```python
from build123d import *

# Parameters (mm, degrees)
SKETCH1_W                      = 98
SKETCH1_H                      = 99
MAIN_BODY_DEPTH                = 1
SKETCH2_R                      = 1.75
FRONTBACKBOLTHOLES_DEPTH       = 2
SKETCH3_R                      = 1.75
SIDEBOLTHOLES_DEPTH            = 2
SKETCH7_W                      = 9
SKETCH7_H                      = 13.5
CUT_EXTRUDE3_DEPTH             = 2
FILLET1_R                      = 4
BOSS_EXTRUDE4_DEPTH            = 2
CAMERAVIEWHOLE_DEPTH           = 4
M3X0_5_TAPPED_HOLE1_D          = 2.5
M3X0_5_TAPPED_HOLE1_DEPTH      = 7.5
M3X0_5_TAPPED_HOLE1_TIP        = 0.751075774
SKETCH16_R                     = 1
WIREPASSTHROUGHS_DEPTH         = 4
SKETCH17_R                     = 2.05
NOTSUREIFNEEDPASSTHROUGH_DEPTH = 4


with BuildPart() as part:
    # Sketch1 → Main Body (new body)
    with BuildSketch(Plane.XY):
        with Locations((49, 49.5)):
            Rectangle(SKETCH1_W, SKETCH1_H)
    extrude(amount=MAIN_BODY_DEPTH)

    # Sketch2 → FrontBackBoltHoles (cut, through all)
    with BuildSketch(Plane.XY.offset(1)):
        with Locations((4, 82)):
            Circle(SKETCH2_R)
        with Locations((94, 82)):
            Circle(SKETCH2_R)
        with Locations((94, 17)):
            Circle(SKETCH2_R)
        with Locations((4, 17)):
            Circle(SKETCH2_R)
    extrude(amount=-FRONTBACKBOLTHOLES_DEPTH, mode=Mode.SUBTRACT)

    # Sketch3 → SideBoltHoles (cut, through all)
    with BuildSketch(Plane.XY.offset(1)):
        with Locations((21, 96)):
            Circle(SKETCH3_R)
        with Locations((77, 96)):
            Circle(SKETCH3_R)
        with Locations((77, 3)):
            Circle(SKETCH3_R)
        with Locations((21, 3)):
            Circle(SKETCH3_R)
    extrude(amount=-SIDEBOLTHOLES_DEPTH, mode=Mode.SUBTRACT)

    # Sketch7 → Cut-Extrude3 (cut, through all)
    with BuildSketch(Plane.XY.offset(1)):
        with Locations((4.5, 92.25)):
            Rectangle(SKETCH7_W, SKETCH7_H)
        with Locations((93.5, 92.25)):
            Rectangle(SKETCH7_W, SKETCH7_H)
        with Locations((93.5, 6.75)):
            Rectangle(SKETCH7_W, SKETCH7_H)
        with Locations((4.5, 6.75)):
            Rectangle(SKETCH7_W, SKETCH7_H)
    extrude(amount=-CUT_EXTRUDE3_DEPTH, mode=Mode.SUBTRACT)

    # Fillet1
    fillet1_edges = [part.edges().sort_by_distance(p)[0] for p in [
        (89, 85.5, 0.5),
        (9, 13.5, 0.5),
        (89, 13.5, 0.5),
        (9, 85.5, 0.5),
    ]]
    fillet(fillet1_edges, radius=FILLET1_R)

    # Sketch15 → Boss-Extrude4 (add)
    with BuildSketch(Plane(origin=(0, 0, 0), x_dir=(-1, 0, 0), z_dir=(0, 0, -1))):
        with BuildLine():
            Line((-22.5, 93.5), (-75.5, 93.5))
            ThreePointArc((-75.5, 93.5), (-86.106601718, 89.106601718), (-90.5, 78.5))
            Line((-90.5, 78.5), (-90.5, 20.5))
            ThreePointArc((-90.5, 20.5), (-86.106601718, 9.893398282), (-75.5, 5.5))
            Line((-75.5, 5.5), (-22.5, 5.5))
            ThreePointArc((-22.5, 5.5), (-11.893398282, 9.893398282), (-7.5, 20.5))
            Line((-7.5, 20.5), (-7.5, 78.5))
            ThreePointArc((-7.5, 78.5), (-11.893398282, 89.106601718), (-22.5, 93.5))
        make_face()
        with BuildLine():
            Line((-35.5, 90.5), (-62.5, 90.5))
            ThreePointArc((-62.5, 90.5), (-80.17766953, 83.17766953), (-87.5, 65.5))
            Line((-87.5, 65.5), (-87.5, 33.5))
            ThreePointArc((-87.5, 33.5), (-80.17766953, 15.82233047), (-62.5, 8.5))
            Line((-62.5, 8.5), (-35.5, 8.5))
            ThreePointArc((-35.5, 8.5), (-17.82233047, 15.82233047), (-10.5, 33.5))
            Line((-10.5, 33.5), (-10.5, 65.5))
            ThreePointArc((-10.5, 65.5), (-17.82233047, 83.17766953), (-35.5, 90.5))
        make_face(mode=Mode.SUBTRACT)
    extrude(amount=BOSS_EXTRUDE4_DEPTH)

    # Sketch10 → CameraViewHole (cut, through all)
    with BuildSketch(Plane.XY.offset(1)):
        with BuildLine():
            Line((40, 35.5), (40, 63.5))
            ThreePointArc((40, 63.5), (49, 72.5), (58, 63.5))
            Line((58, 63.5), (58, 35.5))
            ThreePointArc((58, 35.5), (49, 26.5), (40, 35.5))
        make_face()
    extrude(amount=-CAMERAVIEWHOLE_DEPTH, mode=Mode.SUBTRACT)

    # M3x0.5 Tapped Hole1
    with Locations(Plane.XY.offset(1)):
        with Locations((84, 14.5), (14, 14.5), (14, 84.5), (84, 84.5)):
            Hole(M3X0_5_TAPPED_HOLE1_D / 2, depth=M3X0_5_TAPPED_HOLE1_DEPTH)
            with Locations((0, 0, -(M3X0_5_TAPPED_HOLE1_DEPTH + M3X0_5_TAPPED_HOLE1_TIP / 2))):  # 118° drill point
                Cone(0, M3X0_5_TAPPED_HOLE1_D / 2, M3X0_5_TAPPED_HOLE1_TIP, mode=Mode.SUBTRACT)

    # Sketch16 → WirePassthroughs (cut, through all)
    with BuildSketch(Plane.XY.offset(1)):
        with Locations((27.787, 28.287)):
            Circle(SKETCH16_R)
        with Locations((38.393, 38.893)):
            Circle(SKETCH16_R)
        with Locations((59.607, 60.107)):
            Circle(SKETCH16_R)
        with Locations((70.213, 70.713)):
            Circle(SKETCH16_R)
    extrude(amount=-WIREPASSTHROUGHS_DEPTH, mode=Mode.SUBTRACT)

    # Sketch17 → NotSureIfNeedPassthrough (cut, through all)
    with BuildSketch(Plane.XY.offset(1)):
        with Locations((49, 23.5)):
            Circle(SKETCH17_R)
        with Locations((23, 49.5)):
            Circle(SKETCH17_R)
        with Locations((49, 75.5)):
            Circle(SKETCH17_R)
        with Locations((75, 49.5)):
            Circle(SKETCH17_R)
    extrude(amount=-NOTSUREIFNEEDPASSTHROUGH_DEPTH, mode=Mode.SUBTRACT)


solid = part.part
```
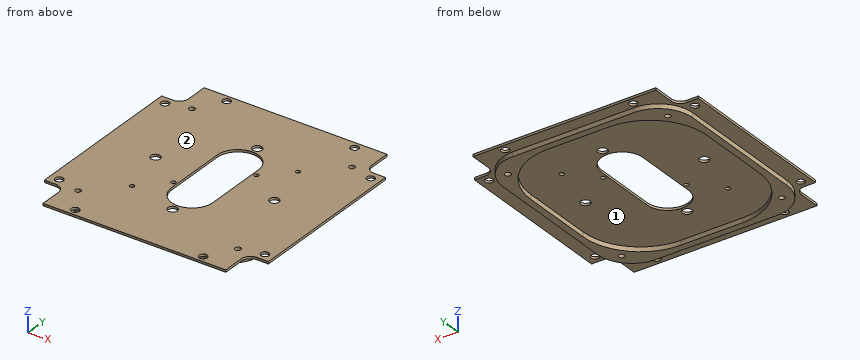
Geometry check sheet. Reference: the model listing, model coordinates, mm. Face numbers are marked on the shaded views. Round coordinates to 2 decimals unless told otherwise and drop trailing zeros. Order: outer loops, then holes, each group sorted by start corner. A loop starts at its lowest first (then second) coordinate and runs counter-clockwise, first axis right, second up. Notation, with made-up numbers: (44, 46.5) -> (57, 46.5) arc R28 cw to (57, 83.5) -> close; hole circle Ø11 at (35.5, -31.75). An arc over 180 degrees is marked (long way). Return JSON: item names as keys, results as strings. Group by question number.
Q1. Section check B-B, the plane x = 49. Record the boundary of the cut face in (y, z).
Q2. Section check A-A, the plane y = 96. Record the boundary of the cut face in (x, z), plus the area to 3 significant figures.
Q3. Material ranges on probe 1 along X at (y, z) = (82, 0.7); probe 2 along Y at (x, z) = (49, 0.2); probe 3 along Y at (x, z) = (4, 0.4), recorded low to high. Write a range as from..to.
Q4. Gauge pin test, flat ends, axial feed: pin 1 (2.5 mm diameter, centred on x = 23, y = 49.5, fed in from -Z); pin 2 (1.6 mm diameter, centred on x = 45.5, z = -1, fed in from -Y); pin 3 (2 mm diameter, centred on x = 63, y = 30.5, fed in from -Z); pin 4 (0.8 mm diameter, centred on x = 2.5, z = 0.5, fed in from +Y). Record the tip position at first contact, or that the pin passes through.
Q5. Section check C-C, the plane y = 49.5. Record the boundary of the cut face in (x, z), plus the area to 3 significant figures.
Q6. Section check D-D, the plane x = 84. Record the boundary of the cut face in (y, z), plus the area to 3 significant figures.
Q7. Release check for a two-part mould opening along X. For the marked faces 1 and 2 record: released by +X, released by -X, zero draft, split by the parting line, or undercut.
Numbers:
{
 "1": {"outline": "(0, 0) -> (5.5, 0) -> (5.5, -2) -> (8.5, -2) -> (8.5, 0) -> (21.45, 0) -> (21.45, 1) -> (0, 1) -> close; (25.55, 0) -> (26.5, 0) -> (26.5, 1) -> (25.55, 1) -> close; (72.5, 0) -> (73.45, 0) -> (73.45, 1) -> (72.5, 1) -> close; (77.55, 0) -> (90.5, 0) -> (90.5, -2) -> (93.5, -2) -> (93.5, 0) -> (99, 0) -> (99, 1) -> (77.55, 1) -> close"},
 "2": {"outline": "(9, 0) -> (19.25, 0) -> (19.25, 1) -> (9, 1) -> close; (22.75, 0) -> (75.25, 0) -> (75.25, 1) -> (22.75, 1) -> close; (78.75, 0) -> (89, 0) -> (89, 1) -> (78.75, 1) -> close", "area": "73.0 mm^2"},
 "3": {"probe 1": "0..2.25, 5.75..92.25, 95.75..98", "probe 2": "0..21.45, 25.55..26.5, 72.5..73.45, 77.55..99", "probe 3": "13.5..15.25, 18.75..80.25, 83.75..85.5"},
 "4": {"pin 1": "through", "pin 2": "y = 5.5", "pin 3": "z = 0", "pin 4": "y = 85.5"},
 "5": {"outline": "(0, 0) -> (7.5, 0) -> (7.5, -2) -> (10.5, -2) -> (10.5, 0) -> (20.95, 0) -> (20.95, 1) -> (0, 1) -> close; (25.05, 0) -> (40, 0) -> (40, 1) -> (25.05, 1) -> close; (58, 0) -> (72.95, 0) -> (72.95, 1) -> (58, 1) -> close; (77.05, 0) -> (87.5, 0) -> (87.5, -2) -> (90.5, -2) -> (90.5, 0) -> (98, 0) -> (98, 1) -> (77.05, 1) -> close", "area": "83.8 mm^2"},
 "6": {"outline": "(0, 0) -> (8.14, 0) -> (8.14, -2) -> (13.25, -2) -> (13.25, 1) -> (0, 1) -> close; (15.75, -2) -> (20.74, -2) -> (20.74, 0) -> (78.26, 0) -> (78.26, -2) -> (83.25, -2) -> (83.25, 1) -> (15.75, 1) -> close; (85.75, -2) -> (90.86, -2) -> (90.86, 0) -> (99, 0) -> (99, 1) -> (85.75, 1) -> close", "area": "134 mm^2"},
 "7": {"face 1": "undercut", "face 2": "zero draft"}
}
